Verification items for the finished model (mm, model axes). A direction names the side the tool comes from. Give positions to 0.01 mm unless a question says otherwise; leave off trailing zeros. Loops run counter-clockwise (first coordinate to the right, second up) from the corner with the lowest first, then second, coordinate; pieces in that order, holes last. Notation, with made-up numbers: M 38,79.25 L 46,79.25 A13 cw 46,102.25 Z; hole C 83.5,-31 d8. An arc over 180 degrees is marked long. Write each question's results on one line, items separated by ' | '. Start each with the question number.
```python
from build123d import *

# Parameters (mm, degrees)
EXTRUDE_1_DEPTH     = 20
SKETCH_2_R          = 2.15
CUT_EXTRUDE_1_DEPTH = 20
SKETCH_3_R          = 1.35
CUT_EXTRUDE_2_DEPTH = 10
FILLET_1_R          = 10
SKETCH_4_R          = 1.35
CUT_EXTRUDE_3_DEPTH = 10


with BuildPart() as part:
    # 스케치1 → 보스-돌출1 (new body)
    with BuildSketch(Plane.XY):
        Polygon((-31.992958445, 23), (-67.5, 2.5), (-87.5, 2.5), (-87.5, -2.5), (77.5, -2.5), (77.5, 2.5), (57.5, 2.5), (21.992958445, 23), (21.992958445, 26), (-31.992958445, 26), align=None)
        Polygon((0.157277926, 2.5), (47.5, 2.5), (11.992958445, 23), align=None, mode=Mode.SUBTRACT)
        Polygon((-16.219455753, 23), (6.219455753, 23), (-5, 3.567332603), align=None, mode=Mode.SUBTRACT)
        Polygon((-21.992958445, 23), (-57.5, 2.5), (-10.157277926, 2.5), align=None, mode=Mode.SUBTRACT)
    extrude(amount=EXTRUDE_1_DEPTH)

    # 스케치2 → 컷-돌출1 (cut)
    with BuildSketch(Plane(origin=(0, 2.5, 0), x_dir=(1, 0, 0), z_dir=(0, 1, 0))):
        with Locations(Location((-77.5, -10, 0), (0, 0, 270))):
            Circle(SKETCH_2_R)
        with Locations(Location((67.5, -10, 0), (0, 0, 270))):
            Circle(SKETCH_2_R)
    extrude(amount=-CUT_EXTRUDE_1_DEPTH, mode=Mode.SUBTRACT)

    # 스케치3 → 컷-돌출2 (cut)
    with BuildSketch(Plane(origin=(0, 26, 0), x_dir=(1, 0, 0), z_dir=(0, 1, 0))):
        with Locations(Location((-25, -5, 0), (0, 0, 270))):
            Circle(SKETCH_3_R)
        with Locations(Location((-25, -15, 0), (0, 0, 270))):
            Circle(SKETCH_3_R)
        with Locations(Location((-5, -5, 0), (0, 0, 270))):
            Circle(SKETCH_3_R)
        with Locations(Location((-5, -15, 0), (0, 0, 270))):
            Circle(SKETCH_3_R)
        with Locations(Location((15, -5, 0), (0, 0, 270))):
            Circle(SKETCH_3_R)
        with Locations(Location((15, -15, 0), (0, 0, 270))):
            Circle(SKETCH_3_R)
    extrude(amount=-CUT_EXTRUDE_2_DEPTH, mode=Mode.SUBTRACT)

    # 필렛1
    fillet_1_edges = [part.edges().sort_by_distance(p)[0] for p in [
        (77.5, 0, 0),
        (77.5, 0, 20),
        (-87.5, 0, 0),
        (-87.5, 0, 20),
    ]]
    fillet(fillet_1_edges, radius=FILLET_1_R - 0.0001)  # a hair under: the kernel refuses the full size

    # 스케치4 → 컷-돌출3 (cut)
    with BuildSketch(Plane.XZ.offset(2.5)):
        with Locations(Location((-65, 15, 0), (0, 0, 270))):
            Circle(SKETCH_4_R)
        with Locations(Location((-65, 5, 0), (0, 0, 270))):
            Circle(SKETCH_4_R)
        with Locations(Location((55, 5, 0), (0, 0, 270))):
            Circle(SKETCH_4_R)
        with Locations(Location((55, 15, 0), (0, 0, 270))):
            Circle(SKETCH_4_R)
        with Locations(Location((-15, 15, 0), (0, 0, 270))):
            Circle(SKETCH_4_R)
        with Locations(Location((5, 15, 0), (0, 0, 270))):
            Circle(SKETCH_4_R)
        with Locations(Location((-15, 5, 0), (0, 0, 270))):
            Circle(SKETCH_4_R)
        with Locations(Location((5, 5, 0), (0, 0, 270))):
            Circle(SKETCH_4_R)
    extrude(amount=-CUT_EXTRUDE_3_DEPTH, mode=Mode.SUBTRACT)


solid = part.part
```
1. Depth check by flat-ended pin: pin 1 Ø2 at (y, z) = (2.5, 8.5) entering from +X; pin 2 Ø3 at (y, z) = (17.5, 9) entering from +X; pin 3 Ø2 at (x, z) = (54.5, 17.5) entering from +Y. Enter the tip coordinate at first touch or a pass-through.
2. Thickness scan on probe 1 along Z at (x, y) = (-65, 2); probe 2 along X at (y, z) = (24.05, 5); probe 3 along X at (y, z) = (-0.3, 10). Record the ranges inside material, lowest first.
3. Set-up check for faces 1 (the face through (-13.661, -0.035, 15.176)), 2 (the face through (21.993, 24, 10)), 3 (the face through (16.339, 23.834, 4.824)), 4 (the face through (-10.531, 13.148, 9.86)): record each of +Z, -Z, +X, -X, +Y, -Y from which the full face is reachable in a straight line by a thin tool's end or side.
4. Section check B-B, the plane x = -34. Record the boundary of the cut face in (y, z).
5. Release check for a two-part mould opening along X. For faces 5 (the face through (65, 2.5, 12)), 6 (the face through (39.995, 12.606, 9.86)), 7 (the face through (-63.661, 1.138, 15.176)) record: released by +X, released by -X, zero draft, split by the parting line, or undercut.
6. Section check D-D, the plane z = 5. State how many separate pieces and enclosed holes the cut face has, plus the area to 3 significant figures.
7. Section check A-A, the plane y = 10.75. Record the boundary of the cut face in (x, z).
8. Section check C-C, the plane x = 15. Record the boundary of the cut face in (y, z), plus the area to 3 significant figures.
Filled sheet:
1) pin 1: x = 77.49 | pin 2: x = 34.12 | pin 3: y = 4.81
2) probe 1: 0 to 3.65, 6.35 to 13.65, 16.35 to 20 | probe 2: -31.99 to -26.35, -23.65 to -6.35, -3.65 to 13.65, 16.35 to 21.99 | probe 3: -87.5 to -79.65, -75.35 to 65.35, 69.65 to 77.5
3) face 1: -Y | face 2: +Z, -Z, +X, +Y | face 3: +Y | face 4: +Z, -Z
4) outline: M -2.5,0 L 2.5,0 L 2.5,20 L -2.5,20 Z; M 16.07,0 L 21.84,0 L 21.84,20 L 16.07,20 Z
5) face 5: zero draft | face 6: released by +X | face 7: undercut
6) separate pieces: 5 | enclosed holes: 0 | area: 1,520 mm2
7) outline: M -53.21,0 L -43.21,0 L -43.21,20 L -53.21,20 Z; M -14.92,0 L -9.15,0 L -9.15,20 L -14.92,20 Z; M -0.85,0 L 4.92,0 L 4.92,20 L -0.85,20 Z; M 33.21,0 L 43.21,0 L 43.21,20 L 33.21,20 Z
8) outline: M -2.5,0 L 2.5,0 L 2.5,20 L -2.5,20 Z; M 21.26,0 L 26,0 L 26,3.65 L 21.26,3.65 Z; M 21.26,6.35 L 26,6.35 L 26,13.65 L 21.26,13.65 Z; M 21.26,16.35 L 26,16.35 L 26,20 L 21.26,20 Z | area: 169 mm2
